Verification items for the finished model (mm, model axes). A direction names the side the tool comes from. Round coordinates to 2 decimals unless told otherwise and drop trailing zeros. Order: outer loops, then holes, each group sorted by start corner. A loop starts at its lowest first (then second) coordinate and runs counter-clockwise, first axis right, second up. Notation, with made-up numbers: M 30.25,50 L 48.25,50 A7 ccw 48.25,56 Z; hole C 20,84 d4. An arc over 180 degrees is marked long. Use CSV: the item, a comma, the result in double quotes. Start each with the question number.
Q1. Set-up check for faces 4 (the face through (38, -19, -1)), 5 (the face through (40.47, 1.01, -1.77)), 6 (the face through (71, -20, 0.5)), 7 (the face through (11, -19, 0)), 8 (the face through (40, 1, 0)): record each of +Z, -Z, +X, -X, +Y, -Y from which the full face is reachable in a straight line by a thin tool's end or side.
Q2. Sectioned sample at D-D (x = 59.5). Enter the section's corners in (y, z).
Q3. Sectioned sample at A-A (x = 50.5). Enter the section's corners in (y, z).
Q4. Sectioned sample at C-C (x = 30.5). Enter the section's corners in (y, z), and give its area (3 significant figures).
Q5. Sectioned sample at B-B (y = -4). State how many separate pieces and enclosed holes the cut face has, and give its area (3 significant figures).
Q6. Gauge pin test, flat ends, axial feed: pin 1 Ø4 at (x, y) = (18.5, -23.5) entering from -Z; pin 2 Ø8 at (x, y) = (70.5, -31.248) entering from -Z; pin 3 Ø6.5 at (x, y) = (50.5, -31.248) entering from -Z; pin 4 Ø0.6 at (y, z) = (-14.5, -0.5) entering from -X. Record the tip position at first contact, or that the pin passes through.
Q7. Scan lines: line 1 (Y direction, x = 50.5, z = 0.25); line 2 (Z direction, x = 54.5, y = -37.5); line 3 (Z direction, x = 77, y = -23). Record each from-to range of solid material in increasing order.
Q8. Mould release check, pull along Y, two halves, no side actions. Record for faces 1 (the face through (70.175, -33.727, 1.24)), 2 (the face through (23, -19, -1)), 3 (the face through (40, -41.25, -1)): +Y half, -Y half, draft (parallel to the pull), parting line (faces both ways), or undercut.
Autodesk Inventor part; units mm, degrees
ref_plane "YZ Plane" through (0, 0, 0) normal (1, 0, 0) x (0, 1, 0)
ref_plane "XZ Plane" through (0, 0, 0) normal (0, 1, 0) x (-1, 0, 0)
ref_plane "XY Plane" through (0, 0, 0) normal (0, 0, 1) x (1, 0, 0)
sketch "Sketch1" plane through (0, 0, 0) normal (0, 0, 1) x (1, 0, 0)
  line L0 (0, 0) -> (81, 0)
  line L1 (0, 0) -> (0, -41.25)
  line L2 (0, -41.25) -> (81, -41.25)
  line L3 (81, -41.25) -> (81, 0)
  line L4 (23, 0) -> (23, 2)
  line L5 (23, 2) -> (38, 2)
  line L6 (38, 2) -> (38, 0)
  line L7 (3, 0) -> (3, -41.25)
  line L8 (18, 0) -> (18, -41.25)
  line L9 (23, 0) -> (23, -41.25)
  line L10 (38, 0) -> (38, -41.25)
  line L11 (43, 0) -> (43, -41.25)
  line L12 (58, 0) -> (58, -41.25)
  line L13 (63, 0) -> (63, -41.25)
  line L14 (78, 0) -> (78, -41.25)
  line L15 (0, 0) -> (3, 0)
  line L16 (3, 0) -> (3, -41.25)
  line L17 (3, -41.25) -> (0, -41.25)
  line L18 (0, -41.25) -> (0, 0)
  line L19 (78, 0) -> (81, 0)
  line L20 (81, 0) -> (81, -41.25)
  line L21 (81, -41.25) -> (78, -41.25)
  line L22 (78, -41.25) -> (78, 0)
  circle A0 centre (10.5, -5.25) radius 2.5
  circle A1 centre (10.5, -31.248) radius 2.5
  circle A2 centre (30.5, -3.25) radius 2.5
  circle A3 centre (30.5, -29.248) radius 2.5
  circle A4 centre (50.5, -5.25) radius 2.5
  circle A5 centre (50.5, -31.248) radius 2.5
  circle A6 centre (70.5, -5.25) radius 2.5
  circle A7 centre (70.5, -31.248) radius 2.5
  point P0 (10.5, -41.25)
  point P1 (50.5, 0)
  point P2 (70.5, 0)
  point P3 (30.5, 0)
  dimension "d0" = 81
  dimension "d2" = 41.25
  dimension "d3" = 2
  dimension "d24" = 5
  dimension "d25" = 5
  dimension "d26" = 5
  dimension "d27" = 5
  dimension "d28" = 5
  dimension "d29" = 5
  dimension "d30" = 5
  dimension "d31" = 5
sketch "Sketch3" plane through (0, 0, 0) normal (0, 1, 0) x (-1, 0, 0)
  line L0 (0, 0) -> (-81, 0)
  line L1 (-23, 0) -> (-38, 0)
  line L2 (0, 0) -> (-81, 0)
  line L3 (-23, 0) -> (-23, -2)
  line L4 (-23, -2) -> (-38, -2)
  line L5 (-38, -2) -> (-38, 0)
  line L6 (-43, 0) -> (-43, 1)
  line L7 (-43, 1) -> (-58, 1)
  line L8 (-58, 1) -> (-58, 0)
  line L9 (-63, 0) -> (-63, 2)
  line L10 (-63, 2) -> (-78, 2)
  line L11 (-78, 2) -> (-78, 0)
  line L12 (-23, -2) -> (-38, -2)
  line L13 (-38, -2) -> (-38, -3.5)
  line L14 (-38, -3.5) -> (-23, -3.5)
  line L15 (-23, -3.5) -> (-23, -2)
  line L16 (-18, 0) -> (-23, -3.5)
  line L17 (-38, -3.5) -> (-43, 0)
  line L18 (-43, 1) -> (-58, 1)
  line L19 (-58, 1) -> (-58, -0.5)
  line L20 (-58, -0.5) -> (-43, -0.5)
  line L21 (-43, -0.5) -> (-43, 1)
  line L22 (-38, 0) -> (-43, 1)
  line L23 (-63, 2) -> (-78, 2)
  line L24 (-78, 2) -> (-78, 0.5)
  line L25 (-78, 0.5) -> (-63, 0.5)
  line L26 (-63, 0.5) -> (-63, 2)
  line L27 (-58, 1) -> (-63, 2)
  line L28 (-58, -0.5) -> (-63, 0.5)
  line L29 (-78, 2) -> (-81, 2)
  line L30 (-81, 2) -> (-78, 0.5)
  line L31 (-43, 1) -> (-38, 0)
  line L32 (-43, 0) -> (-43, 1)
  line L33 (-43, 0) -> (-38, 0)
  line L34 (-38, 0) -> (-43, 1)
  line L35 (-43, 1) -> (-43, 0)
  line L36 (-38, -3.5) -> (-43, -0.5)
  line L37 (-43, -0.5) -> (-58, -0.5)
  line L38 (-58, 1) -> (-58, -0.5)
  line L39 (-58, 1) -> (-43, 1)
  line L40 (-58, -0.5) -> (-58, 1)
  line L41 (-58, 1) -> (-63, 2)
  line L42 (-63, 2) -> (-63, 0.5)
  line L43 (-63, 0.5) -> (-58, -0.5)
  line L44 (-58, -0.5) -> (-60.5, 0)
  line L45 (-58, -0.5) -> (-58, 0)
  line L46 (-58, 0) -> (-60.5, 0)
  line L47 (-60.5, 0) -> (-63, 0.5)
  line L48 (-63, 0.5) -> (-63, 2)
  line L49 (-63, 2) -> (-58, 1)
  line L50 (-58, 1) -> (-58, -0.5)
  point P0 (-3, 0)
  dimension "d4" = 2
  dimension "d5" = 1
  dimension "d6" = 2
  dimension "d7" = 15
  dimension "d8" = 90
  dimension "d11" = 1.5
  dimension "d16" = 15
  dimension "d17" = 1.5
extrude "Extrusion1" add sketch "Sketch1" against normal blind 1.5 contours L0 L7 L2 L1 | L0 L8 L2 L7 | L0 L9 L2 L8 | A0 | A1
extrude "Extrusion2" add sketch "Sketch3" against normal blind 41.25 contours L16 L15 L3 L0 | L14 L13 L4 L15 | L5 L13 L17 L0
extrude "Extrusion3" add sketch "Sketch3" along normal blind 2 contours L16 L15 L3 L0 | L14 L13 L4 L15 | L5 L13 L17 L0
extrude "Extrusion4" add sketch "Sketch3" against normal blind 41.25 contours L0 L6 L22 | L36 L21 L17 | L21 L20 L19 L0 | L0 L8 L7 L6 | L9 L25 L11 L10 | L11 L30 L29
extrude "Extrusion5" add sketch "Sketch3" against normal blind 41.25 contours L19 L28 L0 | L0 L28 L9 L27 L8
extrude "Extrusion6" cut sketch "Sketch1" along normal through all both and the other way through all contours A0 | A1 | A2 | A3 | A4 | A5 | A6 | A7
properties part number "Finger_Support_base_Screwing"
Verdict:
1,face 4,"+Z, +Y, -Y"
1,face 5,"-Z, +X, +Y"
1,face 6,"-Z, +X, +Y, -Y"
1,face 7,"+Z, -X, +Y, -Y"
1,face 8,"+Z, +X, -X, +Y"
2,outline,"M -41.25,-0.2 L 0,-0.2 L 0,1.3 L -41.25,1.3 Z"
3,outline,"M -41.25,-0.5 L -33.75,-0.5 L -33.75,1 L -41.25,1 Z; M -28.75,-0.5 L -7.75,-0.5 L -7.75,1 L -28.75,1 Z; M -2.75,-0.5 L 0,-0.5 L 0,1 L -2.75,1 Z"
4,outline,"M -41.25,-3.5 L -31.75,-3.5 L -31.75,-2 L -41.25,-2 Z; M -26.75,-3.5 L -5.75,-3.5 L -5.75,-2 L -26.75,-2 Z; M -0.75,-3.5 L 2,-3.5 L 2,-2 L -0.75,-2 Z"
4,area,"49.9 mm²"
5,separate pieces,"5"
5,enclosed holes,"0"
5,area,"100 mm²"
6,pin 1,"stops at z = -1.75"
6,pin 2,"stops at z = 0.5"
6,pin 3,"stops at z = -0.5"
6,pin 4,"stops at x = 0"
7,line 1,"y = -41.25 to -33.75, -28.75 to -7.75, -2.75 to 0"
7,line 2,"z = -0.5 to 1"
7,line 3,"z = 0.5 to 2"
8,face 1,"undercut"
8,face 2,"draft"
8,face 3,"-Y half"
